from build123d import *

# Parameters (mm, degrees)
SKETCH1_W               = 200
SKETCH1_H               = 100
BOSS_EXTRUDE1_DEPTH     = 2.5
SKETCH2_W               = 16
SKETCH2_H               = 3.950426225
SKETCH2_H_2             = 3.900095421
SKETCH2_H_3             = 4
BOSS_EXTRUDE2_DEPTH     = 35
CUT_EXTRUDE1_DEPTH      = 39
CUT_EXTRUDE1_DEPTH_BACK = 67
SKETCH3_R               = 6.5
CUT_EXTRUDE2_DEPTH      = 17
FILLET1_R               = 5
SKETCH5_W               = 40.815497855
SKETCH5_H               = 100
CUT_EXTRUDE3_DEPTH      = 17
FILLET2_R               = 5
CHAMFER1_SIZE           = 30
FILLET3_R               = 5
FILLET4_R               = 5
SKETCH6_W               = 47.289599934
SKETCH6_H               = 55
BOSS_EXTRUDE3_DEPTH     = 20
SKETCH7_W               = 39.289599934
SKETCH7_H               = 4
CUT_EXTRUDE4_DEPTH      = 63
FILLET5_R               = 5
SKETCH8_R               = 1.5
CUT_EXTRUDE5_DEPTH      = 63
SKETCH9_W               = 35.271425717
SKETCH9_H               = 49.717701143
CUT_EXTRUDE6_DEPTH      = 12


with BuildPart() as part:
    # Sketch1 → Boss-Extrude1 (new body)
    with BuildSketch(Plane(origin=(0, 0, 0), x_dir=(1, 0, 0), z_dir=(0, 1, 0))):
        Rectangle(SKETCH1_W, SKETCH1_H)
    extrude(amount=BOSS_EXTRUDE1_DEPTH)

    # Sketch2 → Boss-Extrude2 (add)
    with BuildSketch(Plane(origin=(0, 0, 0), x_dir=(-1, 0, 0), z_dir=(0, -1, 0))):
        with Locations((75.379396221, 11.811738969)):
            Rectangle(SKETCH2_W, SKETCH2_H)
        with Locations((75.379396221, -12.263000209)):
            Rectangle(SKETCH2_W, SKETCH2_H_2)
        with Locations((33.379396221, 45.286952081)):
            Rectangle(SKETCH2_W, SKETCH2_H_3)
        with Locations((33.379396221, -45.713047919)):
            Rectangle(SKETCH2_W, SKETCH2_H_3)
    extrude(amount=BOSS_EXTRUDE2_DEPTH)

    # Sketch3 → Cut-Extrude1 (cut, two sides: drawn at the far end of the back side and taken through both)
    with BuildSketch(Plane(origin=(0, 0, -13.786952081), x_dir=(-1, 0, 0), z_dir=(0, 0, -1)).offset(-CUT_EXTRUDE1_DEPTH_BACK)):
        with Locations(Location((33.379396221, -26.491201538, 0), (0, 0, 180))):
            Circle(SKETCH3_R)
        with Locations(Location((75.379396221, -26.491201538, 0), (0, 0, 180))):
            Circle(SKETCH3_R)
    extrude(amount=CUT_EXTRUDE1_DEPTH + CUT_EXTRUDE1_DEPTH_BACK, mode=Mode.SUBTRACT)

    # Sketch4 → Cut-Extrude2 (cut)
    with BuildSketch(Plane(origin=(0, 0, 0), x_dir=(-1, 0, 0), z_dir=(0, -1, 0))):
        Polygon((44.011079662, 50), (100, 50), (100, 13.786952081), (100, -14.213047919), (100, -50), (44.011079662, -50), (44.011079662, -14.213047919), (83.379396221, -14.213047919), (83.379396221, 13.786952081), (44.011079662, 13.786952081), align=None)
    extrude(amount=-CUT_EXTRUDE2_DEPTH, mode=Mode.SUBTRACT)

    # Fillet1
    fillet1_edges = [part.edges().sort_by_distance(p)[0] for p in [
        (-83.379396221, -35, -11.811738968),
        (-67.379396221, -35, -11.811738968),
        (-83.379396221, -35, 12.263000209),
        (-67.379396221, -35, 12.263000209),
        (-41.379396221, -35, -45.286952081),
        (-25.379396221, -35, -45.286952081),
        (-41.379396221, -35, 45.713047919),
        (-25.379396221, -35, 45.713047919),
    ]]
    fillet(fillet1_edges, radius=FILLET1_R)

    # Sketch5 → Cut-Extrude3 (cut)
    with BuildSketch(Plane.XZ):
        with Locations((79.592251073, 0)):
            Rectangle(SKETCH5_W, SKETCH5_H)
    extrude(amount=-CUT_EXTRUDE3_DEPTH, mode=Mode.SUBTRACT)

    # Fillet2
    fillet2_edges = [part.edges().sort_by_distance(p)[0] for p in [
        (-44.011079662, 1.25, -13.786952081),
        (-44.011079662, 1.25, 14.213047919),
    ]]
    fillet(fillet2_edges, radius=FILLET2_R)

    # Chamfer1
    chamfer1_edges = [part.edges().sort_by_distance(p)[0] for p in [
        (59.184502145, 1.25, -50),
        (59.184502145, 1.25, 50),
    ]]
    chamfer(chamfer1_edges, length=CHAMFER1_SIZE)

    # Fillet3
    # the kernel refuses this fillet: 5 mm, written as the material it takes off along each edge
    with BuildSketch(Plane(origin=(-83.379396221, 2.5, -26.286952081), x_dir=(1, 0, 0), z_dir=(0, 0, 1))) as fillet3_piece_1:
        with BuildLine():
            CenterArc((FILLET3_R, -FILLET3_R), FILLET3_R, 90, 90)
            Line((0, -FILLET3_R), (0, 0))
            Line((0, 0), (FILLET3_R, 0))
        make_face()
    extrude(amount=53, mode=Mode.SUBTRACT)

    # Fillet4
    fillet4_edges = [part.edges().sort_by_distance(p)[0] for p in [
        (-67.379396221, 0, -11.811738968),
        (-67.379396221, 0, 12.263000209),
    ]]
    fillet(fillet4_edges, radius=FILLET4_R)

    # Sketch6 → Boss-Extrude3 (add)
    with BuildSketch(Plane.XZ):
        with Locations((15.469477867, -7.508196086)):
            Rectangle(SKETCH6_W, SKETCH6_H)
    extrude(amount=BOSS_EXTRUDE3_DEPTH)

    # Sketch7 → Cut-Extrude4 (cut)
    with BuildSketch(Plane(origin=(0, 0, -35.008196086), x_dir=(-1, 0, 0), z_dir=(0, 0, -1))):
        with Locations((-15.469477867, -18)):
            Rectangle(SKETCH7_W, SKETCH7_H)
    extrude(amount=-CUT_EXTRUDE4_DEPTH, mode=Mode.SUBTRACT)

    # Fillet5
    # the kernel refuses this fillet: 5 mm, written as the material it adds along each edge
    with BuildSketch(Plane(origin=(-4.1753221, -16, -35.008196086), x_dir=(1, 0, 0), z_dir=(0, 0, 1))) as fillet5_piece_1:
        with BuildLine():
            CenterArc((4.898979486, -5), FILLET5_R, 90, 78.463040967)
            Line((0, -4), (-0.09797959, -3.98))
            ThreePointArc((-0.09797959, -3.98), (-0.1, -2), (-0.1, 0))
            Line((-0.1, 0), (0, 0.1))
            Line((0, 0.1), (4.898979486, 0.1))
            Line((4.898979486, 0.1), (4.898979486, 0))
        make_face()
    extrude(amount=55)
    with BuildSketch(Plane(origin=(35.114277834, -16, -35.008196086), x_dir=(-1.570299446029318e-12, -1.0, 0), z_dir=(0, 0, 1))) as fillet5_piece_2:
        with BuildLine():
            CenterArc((5, -4.898979486), FILLET5_R, 101.536959033, 78.463040967)
            Line((0, -4.898979486), (-0.1, -4.898979486))
            Line((-0.1, -4.898979486), (-0.1, 0))
            Line((-0.1, 0), (0, 0.1))
            ThreePointArc((0, 0.1), (2, 0.1), (3.98, 0.09797959))
            Line((3.98, 0.09797959), (4, 0))
        make_face()
    extrude(amount=55)

    # Sketch8 → Cut-Extrude5 (cut)
    with BuildSketch(Plane(origin=(39.114277834, 0, 0), x_dir=(0, 0, -1), z_dir=(1, 0, 0))):
        with Locations((-9.991803914, -15)):
            Circle(SKETCH8_R)
        with Locations((10.008196086, -15)):
            Circle(SKETCH8_R)
        with Locations((0.008196086, -15)):
            Circle(SKETCH8_R)
        with Locations((20.008196086, -15)):
            Circle(SKETCH8_R)
        with Locations((30.008196086, -15)):
            Circle(SKETCH8_R)
    extrude(amount=-CUT_EXTRUDE5_DEPTH, mode=Mode.SUBTRACT)

    # Sketch9 → Cut-Extrude6 (cut)
    with BuildSketch(Plane(origin=(0, 2.5, 0), x_dir=(1, 0, 0), z_dir=(0, 1, 0))):
        with Locations((11.669671686, 7.37138384)):
            Rectangle(SKETCH9_W, SKETCH9_H)
    extrude(amount=-CUT_EXTRUDE6_DEPTH, mode=Mode.SUBTRACT)


solid = part.part
Could you check a few things on this model? Use its own coordinates, in mm. A direction names the side the tool comes from. Coordinates: 2 decimals unless noted, no trailing zeros. Order: outer loops, then holes, each group sorted by start corner. A loop starts at its lowest first (then second) coordinate and runs counter-clockwise, first axis right, second up.
Q1. Suppose I cut it at C-C on x = -19.5. Please give me the cut outline in (y, z).
Q2. Please list where these lines run through material, in increasing order: L1, parallel to Z at x = 19, y = -0.5; L2, parallel to Z at x = 31, y = -15.5; L3, parallel to X at y = -2, z = -27.5.
Q3. Thinking about a two-plate mould opening in X: for faces 1 (the cylindrical face through (-26.81, -33.5, 45.69)), 2 (the flat face through (16, -8, 19.992)), 3 (the cylindrical face through (-27.18, -28.44, -45.26)), which applies, released by +X, released by -X, zero draft, split by the parting line, or undercut?
Q4. Suppose I cut it at D-D on z = 39.5. Please give me the cut outline in (x, y).
Q5. Suppose I cut it at B-B on z = -4.5. Please give me the cut outline in (x, y).
Q6. Will these pins go through, and if not, where does the flat tip stop? pin 1 (2 mm diameter, centred on x = 25.5, z = -21, fed in from +Y); pin 2 (6 mm diameter, centred on y = -21.5, z = 19, fed in from -X); pin 3 (17.5 mm diameter, centred on x = -36, y = -19.5, fed in from +Z).
Q7. Suppose I cut it at A-A on y = -11.5. Please give me the cut outline in (x, z).
Q8. Which directions (+Z, -Z, +X, -X, +Y, -Y) give clear straight access to the entire face, cutting with the end or side of a thin tool? Please do faces 4 (the flat face through (-74, -12, -13.787)), 5 (the flat face through (16, -8, -35.008)), 6 (the cylindrical face through (15.801, -13.513, -9.813)), 7 (the flat face through (11, -3, -32.23)), 8 (the flat face through (-74, -12, 14.213)).
Answer:
1. outline: (0, -50) - (2.5, -50) - (2.5, 50) - (0, 50) - close
2. L1: z = -35.01 to -32.23, 17.49 to 19.99
2. L2: z = -35.01 to -31.42, -28.59 to -21.42, -18.59 to -11.42, -8.59 to -1.42, 1.41 to 8.58, 11.41 to 19.99
2. L3: x = -8.18 to -5.97, 29.31 to 39.11
3. face 1: released by +X
3. face 2: zero draft
3. face 3: undercut
4. outline: (-44.01, 0) - (39.68, 0) - (39.68, 2.5) - (-44.01, 2.5) - close
5. outline: (-82.71, 0) - (-8.18, 0) - (-8.18, -20) - (-4.18, -20) arc R5 cw to (0.72, -16) - (30.22, -16) arc R5 cw to (35.11, -20) - (39.11, -20) - (39.11, 0) - (59.18, 0) - (59.18, 2.5) - (29.31, 2.5) - (29.31, -9.5) - (-5.97, -9.5) - (-5.97, 2.5) - (-78.38, 2.5) arc R5 ccw to start
6. pin 1: stops at y = -9.5
6. pin 2: stops at x = -8.18
6. pin 3: stops at z = 47.71
7. outline: (-83.38, -13.79) - (-67.38, -13.79) - (-67.38, -9.84) - (-83.38, -9.84) - close; (-83.38, 10.31) - (-67.38, 10.31) - (-67.38, 14.21) - (-83.38, 14.21) - close; (-41.38, -47.29) - (-25.38, -47.29) - (-25.38, -43.29) - (-41.38, -43.29) - close; (-41.38, 43.71) - (-25.38, 43.71) - (-25.38, 47.71) - (-41.38, 47.71) - close; (-8.18, -35.01) - (39.11, -35.01) - (39.11, 19.99) - (-8.18, 19.99) - close
8. face 4: -Z, -X, +Y, -Y
8. face 5: -Z, +X, -X, -Y
8. face 6: +X
8. face 7: +Y
8. face 8: +Z, -X, +Y, -Y
